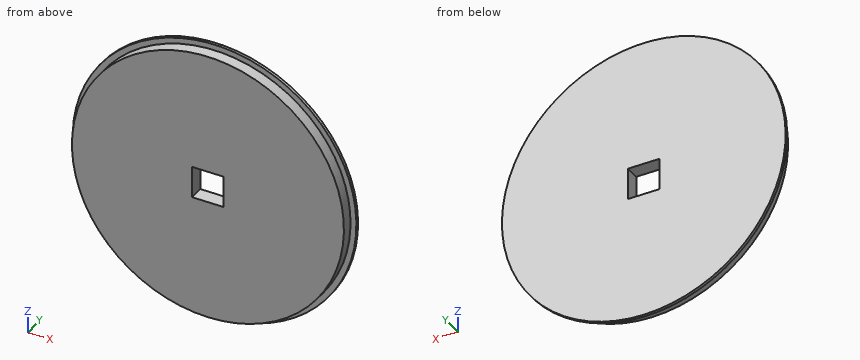
from build123d import *

# Parameters (mm, degrees)
SKETCH2_W          = 6.858
SKETCH2_H          = 6.858
CUT_EXTRUDE1_DEPTH = 44.580249391


with BuildPart() as part:
    # Sketch1 → Revolve1 (revolve)
    with BuildSketch(Plane.XY, mode=Mode.PRIVATE) as revolve1_sk:
        Polygon((0, 3.175), (-30.734, 3.175), (-30.734, 2.54), (-29.464, 2.54), (-29.464, 0), (0, 0), align=None)
    revolve(revolve1_sk.sketch.rotate(Axis((0, 0, 0), (0, 1, 0)), 270), axis=Axis((0, 0, 0), (0, 1, 0)))

    # Sketch2 → Cut-Extrude1 (cut, through all)
    with BuildSketch(Plane(origin=(0, 3.175, 0), x_dir=(1, 0, 0), z_dir=(0, 1, 0))):
        Rectangle(SKETCH2_W, SKETCH2_H)
    extrude(amount=-CUT_EXTRUDE1_DEPTH, mode=Mode.SUBTRACT)


solid = part.part
Here's how the part is built. I have some questions about the finished solid (model axes, mm). Coordinates: 2 decimals unless noted, no trailing zeros. Loops run counter-clockwise (first coordinate to the right, second up) from the corner with the lowest first, then second, coordinate; pieces in that order, holes last.
1. Imagine slicing it at D-D, the plane x = 20. Please give me the cut outline in (y, z) (3 decimals).
2. Imagine slicing it at C-C, the plane y = 1. Please give me the cut outline in (x, z).
3. Imagine slicing it at B-B, the plane z = 0. Please give me the cut outline in (x, y) (3 decimals).
4. For P1, Ø1.5, axis at x = -5, y = 0.5, coming from the -Z side; P2, Ø1, axis at x = -1.5, y = 2.5, coming from the -Z side, each with a flat end and sliding along its axis, tell me the tip position at first contact or that it passes through.
5. I need wall thicknesses on L1, parallel to Z at x = -1, y = 2.75; L2, parallel to X at y = 2.35, z = 0.5; L3, parallel to Y at x = 27.5, z = 13.5 (3 decimals). Which ranges of each line are inside material? Lowest first, please.
6. Imagine slicing it at A-A, the plane x = 0. Please give me the cut outline in (y, z) (3 decimals), and give its area (3 significant figures).
Taken from the geometry:
1. outline: (0, -21.636) - (2.54, -21.636) - (2.54, -23.336) - (3.175, -23.336) - (3.175, 23.336) - (2.54, 23.336) - (2.54, 21.636) - (0, 21.636) - close
2. outline: circle Ø58.93 at (0, 0); hole (-3.43, -3.43) - (3.43, -3.43) - (3.43, 3.43) - (-3.43, 3.43) - close
3. outline: (-30.734, 2.54) - (-29.464, 2.54) - (-29.464, 0) - (-3.429, 0) - (-3.429, 3.175) - (-30.734, 3.175) - close; (3.429, 0) - (29.464, 0) - (29.464, 2.54) - (30.734, 2.54) - (30.734, 3.175) - (3.429, 3.175) - close
4. P1: stops at z = -29.16
4. P2: stops at z = -30.72
5. L1: z = -30.72 to -3.43, 3.43 to 30.72
5. L2: x = -29.46 to -3.43, 3.43 to 29.46
5. L3: y = 2.54 to 3.175
6. outline: (0, -29.464) - (2.54, -29.464) - (2.54, -30.734) - (3.175, -30.734) - (3.175, -3.429) - (0, -3.429) - close; (0, 3.429) - (3.175, 3.429) - (3.175, 30.734) - (2.54, 30.734) - (2.54, 29.464) - (0, 29.464) - close
6. area: 167 mm2
